The figure shows three views and two pictorial views of one solid part (mm, origin at its lowest corner). Answer the questions. A direction names the side the tool comes from. Round coordinates to 2 decimals unless told otherwise and drop trailing zeros. Write each loop counter-clockwise with the first axis right and the second up, starting at its lowest first coordinate (ties: lowest second). Pieces come first, ordered by that corner, then holes.
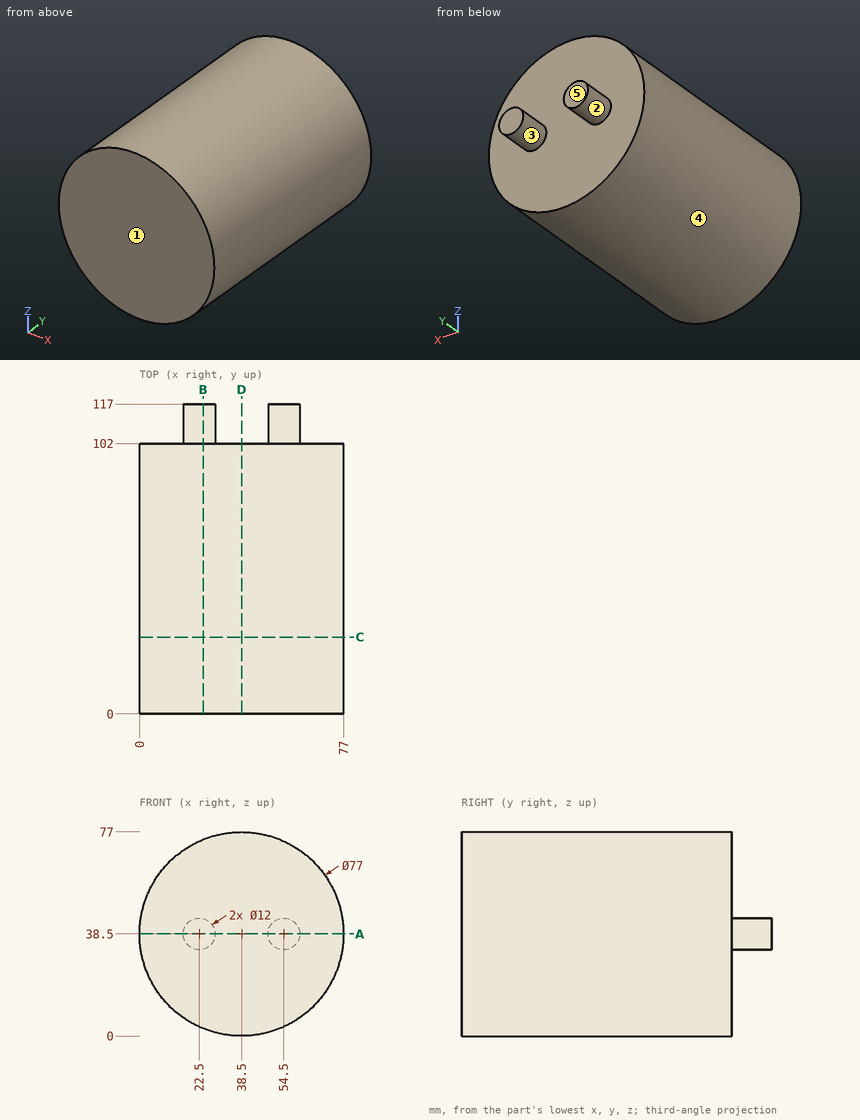
Q1. Flat-ended cylindrical pins translate along their axes: pin 1 Ø3 at (x, z) = (41.5, 44.5) entering from +Y; pin 2 Ø12 at (x, y) = (52, 95.5) entering from +Z; pin 3 Ø2 at (x, y) = (64.5, 58.5) entering from +Z. Find the tip coordinate at first contact, or state that the pin passes through.
Verdict:
pin 1: stops at y = 102
pin 2: stops at z = 76.26
pin 3: stops at z = 67.78
Q2. Section D-D (x = 38.5) is taken. Determine the outline of the cut face in (y, z).
Verdict:
outline: (0, 0) - (102, 0) - (102, 77) - (0, 77) - close
Q3. Straight lines are drawn through the part: probe 1 along Y at (x, z) = (59, 69); probe 2 along X at (y, z) = (53, 64.5); probe 3 along X at (y, z) = (64, 70). For each, find the intervals that lie inside material, in ascending order.
Verdict:
probe 1: y = 0 to 102
probe 2: x = 10.11 to 66.89
probe 3: x = 16.36 to 60.64
Q4. Which of the six approach directions +Z, -Z, +X, -X, +Y, -Y give full straight-line access (tool end or side, diameter ignored) to the marked faces 1 and 2?
Verdict:
face 1: +Z, -Z, +X, -X, -Y
face 2: +Y
Q5. Section B-B (x = 24) is taken. Determine the outline of the cut face in (y, z).
Verdict:
outline: (0, 2.83) - (102, 2.83) - (102, 32.69) - (117, 32.69) - (117, 44.31) - (102, 44.31) - (102, 74.17) - (0, 74.17) - close
Q6. Section C-C (y = 29) is taken. Determine the outline of the cut face in (x, z).
Verdict:
outline: circle Ø77 at (38.5, 38.5)
Q7. Section A-A (z = 38.5) is taken. Determine the outline of the cut face in (x, y), then the cut area to 3 significant figures.
Verdict:
outline: (0, 0) - (77, 0) - (77, 102) - (60.5, 102) - (60.5, 117) - (48.5, 117) - (48.5, 102) - (28.5, 102) - (28.5, 117) - (16.5, 117) - (16.5, 102) - (0, 102) - close
area: 8,210 mm2
Q8. Determine the mould class of the marked faces 3, 4 and 5 for opening direction X: pulls with the +X half, pulls with the -X half, needs draft (parallel to the pull), parting line crosses it, or undercut.
Verdict:
face 3: undercut
face 4: parting line crosses it
face 5: needs draft
